```python
from build123d import *

# Parameters (mm, degrees)
F1_R   = 12
F1_R_2 = 10


with BuildPart() as f2:
    # F2: sweep along a path in F0
    with BuildLine(Plane.XZ) as f2_path:
        Line((-0.000112, -2.6e-05), (-10.000112, -2.6e-05))
        ThreePointArc((-10.000112, -2.6e-05), (-24.142248, -5.85789), (-30.000112, -20.000026))
        Line((-30.000112, -20.000026), (-30.000112, -30.000026))
    # F1 (on Right) → F2 (sweep)
    with BuildSketch(Plane.YZ):
        Circle(F1_R)
        Circle(F1_R_2, mode=Mode.SUBTRACT)
    sweep(path=f2_path.line)


solid = f2.part
```
Build history of the part. All positions in model axes, mm. Coordinates: 2 decimals unless noted, no trailing zeros. Order: outer loops, then holes, each group sorted by start corner. A loop starts at its lowest first (then second) coordinate and runs counter-clockwise, first axis right, second up. Notation, with made-up numbers: M 23.5,33.25 L 54.5,33.25 A29 cw 54.5,67.25 Z; hole C -10.75,34.25 d8. An arc over 180 degrees is marked long. One line per question, with ' | ' between items. Start each with the question number.
1. Flat gauge pins, fed straight in: P1, Ø1, axis at y = 1.5, z = 4, coming from the +X side; P2, Ø2, axis at x = -5.5, z = 7.5, coming from the -Y side; P3, Ø12, axis at x = -21.5, z = -15.5, coming from the +Y side; P4, Ø6, axis at x = -11, z = -16, coming from the +Y side. Where does each tip first touch, or does it go through?
2. Cut at A-A (x = -3.5). Write the cut outline in (y, z), plus the area to 3 significant figures.
3. Wall check: line 1 along Z through (x, y) = (-5.75, 0); line 2 along X through (y, z) = (2.5, -17); line 3 along Z through (x, y) = (-9, -7). Give the ranges that are in metal, low to high. Write a range as [from, to].
4. Mould opens along Y. For faces 1 (the face through (-5.07, -2.17, 9.76)), 2 (the face through (-5.07, -11.99, -0.53)), 3 (the face through (0, -9, -5)) say: +Y half, -Y half, draft (parallel to the pull), parting line (faces both ways), or undercut.
The answers:
1) P1: stops at x = -27.1 | P2: stops at y = -10.09 | P3: stops at y = 11.89 | P4: passes through
2) outline: C 0,0 d24; hole C 0,0 d20 | area: 138 mm2
3) line 1: z = [-12, -10], [10, 12] | line 2: x = [-41.59, -39.53], [-19.87, -17.7] | line 3: z = [-9.75, -7.14], [7.14, 9.75]
4) face 1: undercut | face 2: parting line | face 3: draft
